Check sheet for the modelled part. Datum: model origin and axes. Units: mm. Face numbers are marked on the shaded views. A direction names the side the tool comes from. Give positions to 0.01 mm unless a question says otherwise; leave off trailing zeros. Loops run counter-clockwise (first coordinate to the right, second up) from the corner with the lowest first, then second, coordinate; pieces in that order, holes last. Notation, with made-up numbers: (-15.75, 74) - (19.25, 74) arc R12 cw to (19.25, 91) - close; hole circle Ø2 at (-21, -1). An arc over 180 degrees is marked (long way). Use CSV: the item, a comma, the result in double quotes.
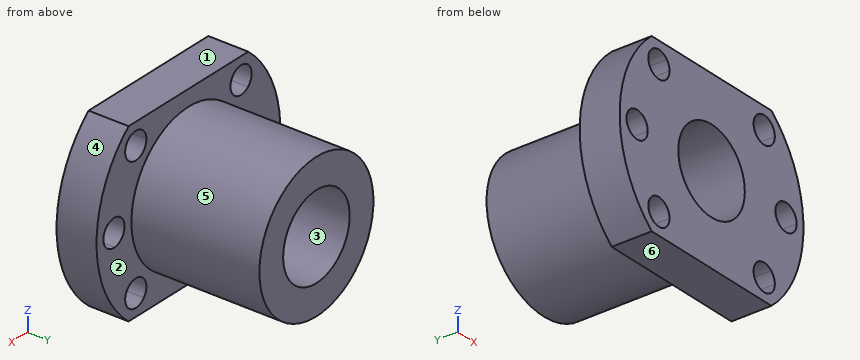
from build123d import *

# Parameters (mm, degrees)
F0_R     = 18
F1_DEPTH = 32
F2_R     = 29
F3_DEPTH = 10
F5_DEPTH = 42


with BuildPart() as f1:
    # F0 (on Front) → F1 (new body)
    with BuildSketch(Plane.XZ):
        Circle(F0_R)
    extrude(amount=F1_DEPTH)

    # F2 (on face) → F3 (join)
    with BuildSketch(Plane.XZ.offset(32)):
        Circle(F2_R)
    extrude(amount=F3_DEPTH)

    # F4 (on face) → F5 (cut)
    with BuildSketch(Plane.XZ.offset(42)):
        with BuildLine():
            Line((0, 0), (-7.4246212025, 7.4246212025))
            ThreePointArc((-7.4246212025, 7.4246212025), (-9.7007350914, 4.0181760398), (-10.5, 0))
            Line((-10.5, 0), (0, 0))
        make_face()
        with BuildLine():
            ThreePointArc((-10.5, 0), (0, -10.5), (10.5, 0))
            ThreePointArc((10.5, 0), (4.0181760398, 9.7007350914), (-7.4246212025, 7.4246212025))
            Line((-7.4246212025, 7.4246212025), (0, 0))
            Line((0, 0), (-10.5, 0))
        make_face()
        with BuildLine():
            Line((-16.6170093579, 16.6170093579), (-14.2482016409, 14.2482016409))
            ThreePointArc((-14.2482016409, 14.2482016409), (-13.522012924, 15.3350198595), (-13.2670093579, 16.6170093579))
            Line((-13.2670093579, 16.6170093579), (-16.6170093579, 16.6170093579))
        make_face()
        with BuildLine():
            ThreePointArc((-18.8109516732, 14.0853859425), (-16.4975450742, 13.2691401423), (-14.2482016409, 14.2482016409))
            Line((-14.2482016409, 14.2482016409), (-16.6170093579, 16.6170093579))
            ThreePointArc((-16.6170093579, 16.6170093579), (-17.7591493316, 15.3903416147), (-18.8109516732, 14.0853859425))
        make_face()
        with BuildLine():
            ThreePointArc((-18.9858170749, 18.9858170749), (-19.9648785735, 16.4975450742), (-18.8109516732, 14.0853859425))
            ThreePointArc((-18.8109516732, 14.0853859425), (-17.7591493316, 15.3903416147), (-16.6170093579, 16.6170093579))
            Line((-16.6170093579, 16.6170093579), (-18.9858170749, 18.9858170749))
        make_face()
        with BuildLine():
            Line((-18.9858170749, 18.9858170749), (-16.6170093579, 16.6170093579))
            ThreePointArc((-16.6170093579, 16.6170093579), (-15.3903416147, 17.7591493316), (-14.0853859425, 18.8109516732))
            ThreePointArc((-14.0853859425, 18.8109516732), (-16.4975450742, 19.9648785735), (-18.9858170749, 18.9858170749))
        make_face()
        with BuildLine():
            ThreePointArc((-23.5, 0), (-23.440229841, 1.675), (-23.2612234043, 3.3414795731))
            ThreePointArc((-23.2612234043, 3.3414795731), (-26.85, 0), (-23.2612234043, -3.3414795731))
            ThreePointArc((-23.2612234043, -3.3414795731), (-23.440229841, -1.675), (-23.5, 0))
        make_face()
        with BuildLine():
            Line((-23.5, 0), (-20.15, 0))
            ThreePointArc((-20.15, 0), (-21.04822497, 2.2828270198), (-23.2612234043, 3.3414795731))
            ThreePointArc((-23.2612234043, 3.3414795731), (-23.440229841, 1.675), (-23.5, 0))
        make_face()
        with BuildLine():
            ThreePointArc((-23.2612234043, -3.3414795731), (-21.04822497, -2.2828270198), (-20.15, 0))
            Line((-20.15, 0), (-23.5, 0))
            ThreePointArc((-23.5, 0), (-23.440229841, -1.675), (-23.2612234043, -3.3414795731))
        make_face()
        with BuildLine():
            ThreePointArc((-14.0853859425, -18.8109516732), (-16.6170093579, -16.6170093579), (-18.8109516732, -14.0853859425))
            ThreePointArc((-18.8109516732, -14.0853859425), (-18.9858170749, -18.9858170749), (-14.0853859425, -18.8109516732))
        make_face()
        with BuildLine():
            ThreePointArc((-13.2670093579, -16.6170093579), (-15.2254646687, -13.5696985142), (-18.8109516732, -14.0853859425))
            ThreePointArc((-18.8109516732, -14.0853859425), (-16.6170093579, -16.6170093579), (-14.0853859425, -18.8109516732))
            ThreePointArc((-14.0853859425, -18.8109516732), (-13.4782645099, -17.7878128338), (-13.2670093579, -16.6170093579))
        make_face()
        with BuildLine():
            ThreePointArc((14.0853859425, -18.8109516732), (16.6170093579, -16.6170093579), (18.8109516732, -14.0853859425))
            ThreePointArc((18.8109516732, -14.0853859425), (14.2482016409, -14.2482016409), (14.0853859425, -18.8109516732))
        make_face()
        with BuildLine():
            ThreePointArc((19.9670093579, -16.6170093579), (19.6643202016, -15.2254646687), (18.8109516732, -14.0853859425))
            ThreePointArc((18.8109516732, -14.0853859425), (16.6170093579, -16.6170093579), (14.0853859425, -18.8109516732))
            ThreePointArc((14.0853859425, -18.8109516732), (17.7878128338, -19.7557542059), (19.9670093579, -16.6170093579))
        make_face()
        with BuildLine():
            ThreePointArc((23.5, 0), (23.440229841, 1.675), (23.2612234043, 3.3414795731))
            ThreePointArc((23.2612234043, 3.3414795731), (20.15, 0), (23.2612234043, -3.3414795731))
            ThreePointArc((23.2612234043, -3.3414795731), (23.440229841, -1.675), (23.5, 0))
        make_face()
        with BuildLine():
            ThreePointArc((26.85, 0), (25.7828270198, 2.45177503), (23.2612234043, 3.3414795731))
            ThreePointArc((23.2612234043, 3.3414795731), (23.440229841, 1.675), (23.5, 0))
            ThreePointArc((23.5, 0), (23.440229841, -1.675), (23.2612234043, -3.3414795731))
            ThreePointArc((23.2612234043, -3.3414795731), (25.7828270198, -2.45177503), (26.85, 0))
        make_face()
        with BuildLine():
            ThreePointArc((19.9670093579, 16.6170093579), (17.7878128338, 19.7557542059), (14.0853859425, 18.8109516732))
            ThreePointArc((14.0853859425, 18.8109516732), (15.3903416147, 17.7591493316), (16.6170093579, 16.6170093579))
            Line((16.6170093579, 16.6170093579), (19.9670093579, 16.6170093579))
        make_face()
        with BuildLine():
            ThreePointArc((16.6170093579, 16.6170093579), (17.7591493316, 15.3903416147), (18.8109516732, 14.0853859425))
            ThreePointArc((18.8109516732, 14.0853859425), (19.6643202016, 15.2254646687), (19.9670093579, 16.6170093579))
            Line((19.9670093579, 16.6170093579), (16.6170093579, 16.6170093579))
        make_face()
        with BuildLine():
            Line((16.6170093579, 16.6170093579), (13.2670093579, 16.6170093579))
            ThreePointArc((13.2670093579, 16.6170093579), (15.2254646687, 13.5696985142), (18.8109516732, 14.0853859425))
            ThreePointArc((18.8109516732, 14.0853859425), (17.7591493316, 15.3903416147), (16.6170093579, 16.6170093579))
        make_face()
        with BuildLine():
            ThreePointArc((14.0853859425, 18.8109516732), (13.4782645099, 17.7878128338), (13.2670093579, 16.6170093579))
            Line((13.2670093579, 16.6170093579), (16.6170093579, 16.6170093579))
            ThreePointArc((16.6170093579, 16.6170093579), (15.3903416147, 17.7591493316), (14.0853859425, 18.8109516732))
        make_face()
        with BuildLine():
            Line((-18.8944436277, 22), (-8.2613558209, 22))
            ThreePointArc((-8.2613558209, 22), (0, 23.5), (8.2613558209, 22))
            Line((8.2613558209, 22), (18.8944436277, 22))
            ThreePointArc((18.8944436277, 22), (0, 29), (-18.8944436277, 22))
        make_face()
        with BuildLine():
            ThreePointArc((8.2613558209, 22), (0, 23.5), (-8.2613558209, 22))
            Line((-8.2613558209, 22), (8.2613558209, 22))
        make_face()
        with BuildLine():
            Line((-8.2613558209, -22), (-18.8944436277, -22))
            ThreePointArc((-18.8944436277, -22), (0, -29), (18.8944436277, -22))
            Line((18.8944436277, -22), (8.2613558209, -22))
            ThreePointArc((8.2613558209, -22), (0, -23.5), (-8.2613558209, -22))
        make_face()
        with BuildLine():
            Line((8.2613558209, -22), (-8.2613558209, -22))
            ThreePointArc((-8.2613558209, -22), (0, -23.5), (8.2613558209, -22))
        make_face()
        with BuildLine():
            Line((-16.6170093579, 16.6170093579), (-13.2670093579, 16.6170093579))
            ThreePointArc((-13.2670093579, 16.6170093579), (-13.4782645099, 17.7878128338), (-14.0853859425, 18.8109516732))
            ThreePointArc((-14.0853859425, 18.8109516732), (-15.3903416147, 17.7591493316), (-16.6170093579, 16.6170093579))
        make_face()
    extrude(amount=-F5_DEPTH, mode=Mode.SUBTRACT)


solid = f1.part
1. Set-up check for the marked faces 1 and 2: record each of +Z, -Z, +X, -X, +Y, -Y from which the full face is reachable in a straight line by a thin tool's end or side.
Completed:
face 1,"+Z, +X, -X, +Y, -Y"
face 2,"+Y"
2. Sectioned sample at A-A, the plane x = 0. Record the boundary of the cut face in (y, z).
Completed:
outline,"(-42, -22) - (-32, -22) - (-32, -18) - (0, -18) - (0, -10.5) - (-42, -10.5) - close; (-42, 10.5) - (0, 10.5) - (0, 18) - (-32, 18) - (-32, 22) - (-42, 22) - close"
3. Sectioned sample at D-D, the plane x = 7.5. Record the boundary of the cut face in (y, z).
Completed:
outline,"(-42, -22) - (-32, -22) - (-32, -16.36) - (0, -16.36) - (0, -7.35) - (-42, -7.35) - close; (-42, 7.35) - (0, 7.35) - (0, 16.36) - (-32, 16.36) - (-32, 22) - (-42, 22) - close"
4. Sectioned sample at C-C, the plane y = -4.5. Record the boundary of the cut face in (x, z).
Completed:
outline,"circle Ø36 at (0, 0); hole circle Ø21 at (0, 0)"
5. Release check for a two-part mould opening along X. For the marked faces 3, 4, 5 and 6 record: released by +X, released by -X, zero draft, split by the parting line, or undercut.
Completed:
face 3,"undercut"
face 4,"released by +X"
face 5,"split by the parting line"
face 6,"zero draft"
6. Sectioned sample at B-B, the plane z = -15. Record the boundary of the cut face in (x, y).
Completed:
outline,"(-24.82, -42) - (-19.55, -42) - (-19.55, -32) - (-24.82, -32) - close; (-13.68, -42) - (13.68, -42) - (13.68, -32) - (9.95, -32) - (9.95, 0) - (-9.95, 0) - (-9.95, -32) - (-13.68, -32) - close; (19.55, -42) - (24.82, -42) - (24.82, -32) - (19.55, -32) - close"
7. Go/stop test with flat-tipped pins: pin 1 Ø4 at (x, y) = (-17.5, -9) entering from -Z; pin 2 Ø2 at (y, z) = (-37, 7.5) entering from +X; pin 3 Ø4 at (x, y) = (8, -21) entering from +Z; pin 4 Ø13 at (x, z) = (13, -5.5) entering from +Y. Record where each tip stops, or that it passes through.
Completed:
pin 1,"stops at z = -9.15"
pin 2,"stops at x = 28.26"
pin 3,"stops at z = 16.97"
pin 4,"stops at y = 0"
8. Scan lines: line 1 along X through (y, z) = (-2, 0.5); line 2 along Z through (x, y) = (-17.5, -37); line 3 along Z through (x, y) = (0, -31). Record each from-to range of solid material in increasing order.
Completed:
line 1,"x = -17.99 to -10.49, 10.49 to 17.99"
line 2,"z = -22 to -19.85, -13.39 to 13.39, 19.85 to 22"
line 3,"z = -18 to -10.5, 10.5 to 18"
